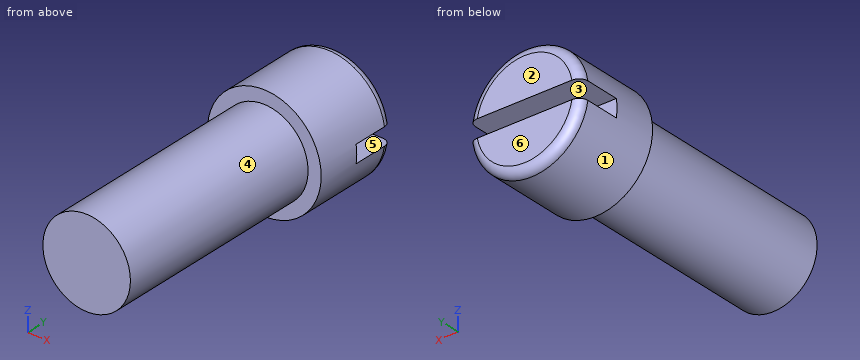
```python
from build123d import *

# Parameters (mm, degrees)
F0_R     = 1.651
F0_R_2   = 1.27
F1_DEPTH = 2.54
F2_DEPTH = 8.89
F3_R     = 0.254
F5_DEPTH = 1.27


with BuildPart() as f1:
    # F0 (on Front) → F1 (new body)
    with BuildSketch(Plane.XZ):
        Circle(F0_R)
        Circle(F0_R_2, mode=Mode.SUBTRACT)
    extrude(amount=F1_DEPTH)

    # F0 (on Front) → F2 (join)
    with BuildSketch(Plane.XZ):
        Circle(F0_R_2)
    extrude(amount=F2_DEPTH)

    # F3
    f3_edges = [f1.edges().sort_by_distance(p)[0] for p in [
        (-1.651, 0, 0),
    ]]
    fillet(f3_edges, radius=F3_R)

    # F4 (on face) → F5 (cut)
    with BuildSketch(Plane.XZ):
        with BuildLine():
            Line((1.6313445375, 0.254), (-1.6313445375, 0.254))
            ThreePointArc((-1.6313445375, 0.254), (-1.651, 0), (-1.6313445375, -0.254))
            Line((-1.6313445375, -0.254), (1.6313445375, -0.254))
            ThreePointArc((1.6313445375, -0.254), (1.651, 0), (1.6313445375, 0.254))
        make_face()
    extrude(amount=F5_DEPTH, mode=Mode.SUBTRACT)


solid = f1.part
```
Source: CAD feature listing. Evaluate the final solid. Frame: model axes, mm. Face numbers are marked on the shaded views. A direction names the side the tool comes from. Coordinates: 2 decimals unless noted, no trailing zeros. Loops run counter-clockwise (first coordinate to the right, second up) from the corner with the lowest first, then second, coordinate; pieces in that order, holes last. Notation, with made-up numbers: M -16.75,-25.75 L 19.25,-25.75 A15 ccw 19.25,-13.75 Z; hole C -33,63.5 d11. An arc over 180 degrees is marked long. Use a Markdown table: item, result. Add a question column.
Q1. Section query D-D, the plane y = -2.25. Return loops of the section in (x, z).
Q2. Draft query along Z for the marked faces 1, 2 and 3. Return one class per face: pulls with the +Z half, pulls with the -Z half, needs draft (parallel to the pull), parting line crosses it, or undercut.
Q3. First-contact query: pin 1 (1 mm diameter, centred on y = -6.5, z = -1, fed in from -X); pin 2 (1 mm diameter, centred on x = 0, y = -4, fed in from +Z). Flat tips, straight axial feed; report the tip coordinate or a pass-through.
Q4. Section query C-C, the plane y = -4.5. Return loops of the section in (x, z).
Q5. Section query A-A, the plane x = 0. Return loops of the section in (y, z).
Q6. Material intervals for L1, parallel to Z at x = -0.6, y = -0.25; L2, parallel to Y at x = -1.4, z = 0.3; L3, parallel to Z at x = 1.5, y = -0.25, sorted ascending.
Q7. Section query B-B, the plane z = 0. Return loops of the section in (x, y), and give its area (3 significant figures).
Q8. Access query for the marked faces 4, 5 and 6. Directions: +Z, -Z, +X, -X, +Y, -Y. A direction counts if a zero-diameter tool reaches every point of the face in a straight line with its end or side. Return the directions, or none.
Result:
| question | item | result |
|---|---|---|
| 1 | outline | C 0,0 d3.3 |
| 2 | face 1 | parting line crosses it |
| 2 | face 2 | needs draft |
| 2 | face 3 | undercut |
| 3 | pin 1 | stops at x = -1.17 |
| 3 | pin 2 | stops at z = 1.27 |
| 4 | outline | C 0,0 d2.54 |
| 5 | outline | M -8.89,-1.27 L -2.54,-1.27 L -2.54,-1.65 L -0.25,-1.65 A0.25 ccw 0,-1.4 L 0,-0.25 L -1.27,-0.25 L -1.27,0.25 L 0,0.25 L 0,1.4 A0.25 ccw -0.25,1.65 L -2.54,1.65 L -2.54,1.27 L -8.89,1.27 Z |
| 6 | L1 | z = -1.54 to -0.25, 0.25 to 1.54 |
| 6 | L2 | y = -2.54 to 0 |
| 6 | L3 | z = -0.69 to -0.25, 0.25 to 0.69 |
| 7 | outline | M -1.65,-2.54 L -1.27,-2.54 L -1.27,-8.89 L 1.27,-8.89 L 1.27,-2.54 L 1.65,-2.54 L 1.65,-1.27 L -1.65,-1.27 Z |
| 7 | area | 20.3 mm2 |
| 8 | face 4 | -Y |
| 8 | face 5 | +X, -X, +Y |
| 8 | face 6 | +Z, -Z, +X, -X, +Y |
